Read the model definition and answer for the solid it produces. Units are mm, in the model's axes. A direction names the side the tool comes from. Round coordinates to 2 decimals unless told otherwise and drop trailing zeros. Order: outer loops, then holes, each group sorted by start corner. A loop starts at its lowest first (then second) coordinate and runs counter-clockwise, first axis right, second up. Notation, with made-up numbers: (-19, -5) - (-5, -5) arc R19 cw to (-5, 20) - close; hole circle Ø5 at (45.5, 54.5). An arc over 180 degrees is marked (long way). Answer as a JSON object with one key per item and string values. Group by question number.
Q1. Given pin 1 Ø3 at (y, z) = (4.5, -9.5) entering from +X; pin 2 Ø2 at (y, z) = (3, -13) entering from +X; pin 3 Ø3 at (x, z) = (0, 0) entering from +Y, each flat-ended and moving along its own axis, determine where each tip first touches the part or whether it passes through.
Q2. A cutting plane is placed at B-B on y = 3.2. Count the separate pieces of the cut face and the enclosed holes in it, and give its area (3 significant figures).
Q3. A tool of negligible diameter and unlimited length cuts with its end or side. For faces 3 (the cylindrical face through (5.77, 2.96, 18.65)), 4 (the cylindrical face through (19.6, 3, -6.9)), 5 (the cylindrical face through (12.32, 3.04, -16.78)), from which of +Z, -Z, +X, -X, +Y, -Y can it reach the whole face along a straight path? Write none if from no direction.
Q4. The mould has two halves that part along X. Classify faces 1 (the flat face through (6, 3, -28)), 2 (the cylindrical face through (11.046, 3.042, 17.717)): pulls with the +X half, pulls with the -X half, needs draft (parallel to the pull), parting line crosses it, or undercut.
Q5. Consider line 1 (Z direction, x = 0, y = 3); line 2 (Z direction, x = 21, y = 4.7); line 3 (X direction, y = 4.1, z = 0). Determine where each line is inside the solid, lowest interval first.
Q6. A cutting plane is placed at C-C on z = -23.5. Determine the outline of the cut face in (x, y), and give its area (3 significant figures).
Q7. A cutting plane is placed at A-A on x = 0. Determine the outline of the cut face in (y, z), and give its area (3 significant figures).
```python
from build123d import *

# Parameters (mm, degrees)
BOSS_EXTRUDE1_DEPTH = 6
BOSS_EXTRUDE2_DEPTH = 6
SKETCH2_R           = 2
CUT_EXTRUDE1_DEPTH  = 7


with BuildPart() as part:
    # Sketch1 → Boss-Extrude1 (new body)
    with BuildSketch(Plane(origin=(0, 0, 0), x_dir=(1, 0, 0), z_dir=(0, 1, 0))):
        with BuildLine():
            Line((5.999994922, -17.000000726), (6.000000976, 32.999999274))
            ThreePointArc((6.000000976, 32.999999274), (3.1827e-05, 38.999972559), (-5.999944142, 33.000006094))
            Line((-5.999944142, 33.000006094), (-5.999994922, -16.999993906))
            ThreePointArc((-5.999994922, -16.999993906), (-3.41e-06, -22.999994922), (5.999994922, -17.000000726))
        make_face()
    extrude(amount=BOSS_EXTRUDE1_DEPTH)

    # Sketch4 → Boss-Extrude2 (add)
    with BuildSketch(Plane(origin=(0, 6, 0), x_dir=(1, 0, 0), z_dir=(0, 1, 0))):
        with BuildLine():
            Line((-2.743025532, 18.19970901), (3.351302477, -22.235567688))
            ThreePointArc((3.351302477, -22.235567688), (3.541272199, -22.468242769), (3.739439393, -22.693977021))
            ThreePointArc((3.739439393, -22.693977021), (4.275797924, -22.599060868), (4.809758376, -22.491470036))
            ThreePointArc((4.809758376, -22.491470036), (5.335701359, -20.15196829), (5.179210857, -17.759188492))
            ThreePointArc((5.179210857, -17.759188492), (6.10970176, -17.460943428), (7.023146788, -17.113982885))
            ThreePointArc((7.023146788, -17.113982885), (8.392641943, -19.082324182), (10.262473747, -20.583528186))
            ThreePointArc((10.262473747, -20.583528186), (10.747026347, -20.334734439), (11.225551479, -20.074535959))
            ThreePointArc((11.225551479, -20.074535959), (11.038548046, -17.683947297), (10.183725752, -15.443598376))
            ThreePointArc((10.183725752, -15.443598376), (10.984968279, -14.884336496), (11.755563092, -14.283547788))
            ThreePointArc((11.755563092, -14.283547788), (13.644394202, -15.760775419), (15.873642273, -16.644142542))
            ThreePointArc((15.873642273, -16.644142542), (16.263334316, -16.263577617), (16.643905071, -15.873891267))
            ThreePointArc((16.643905071, -15.873891267), (15.760571298, -13.644629981), (14.283371923, -11.755776772))
            ThreePointArc((14.283371923, -11.755776772), (14.884172159, -10.985190947), (15.443446026, -10.183956787))
            ThreePointArc((15.443446026, -10.183956787), (17.683782158, -11.038812596), (20.074368023, -11.225851792))
            ThreePointArc((20.074368023, -11.225851792), (20.334573661, -10.747330553), (20.583374658, -10.262781675))
            ThreePointArc((20.583374658, -10.262781675), (19.082198626, -8.392927413), (17.113877817, -7.023402811))
            ThreePointArc((17.113877817, -7.023402811), (17.460852025, -6.109962974), (17.759111009, -5.179476534))
            ThreePointArc((17.759111009, -5.179476534), (20.151888466, -5.336002831), (22.491398079, -4.810094847))
            ThreePointArc((22.491398079, -4.810094847), (22.5989969, -4.276136005), (22.693921077, -3.739778893))
            ThreePointArc((22.693921077, -3.739778893), (20.708288865, -2.395476413), (18.423740564, -1.66696869))
            ThreePointArc((18.423740564, -1.66696869), (18.486058563, -0.691837978), (18.496801044, 0.285222939))
            ThreePointArc((18.496801044, 0.285222939), (20.829411048, 0.840934203), (22.909968714, 2.033060135))
            ThreePointArc((22.909968714, 2.033060135), (22.855400089, 2.575011992), (22.788013017, 3.115519655))
            ThreePointArc((22.788013017, 3.115519655), (20.494356761, 3.814823179), (18.096573111, 3.837582915))
            ThreePointArc((18.096573111, 3.837582915), (17.868697673, 4.787759858), (17.590969135, 5.724579102))
            ThreePointArc((17.590969135, 5.724579102), (19.656149051, 6.943150542), (21.29288809, 8.695568802))
            ThreePointArc((21.29288809, 8.695568802), (21.081000682, 9.197358874), (20.857289998, 9.69399061))
            ThreePointArc((20.857289998, 9.69399061), (18.459411122, 9.686158991), (16.161445721, 9.001148437))
            ThreePointArc((16.161445721, 9.001148437), (15.66362458, 9.84194422), (15.122102421, 10.65528129))
            ThreePointArc((15.122102421, 10.65528129), (16.73635195, 12.428437486), (17.783840917, 14.58543802))
            ThreePointArc((17.783840917, 14.58543802), (17.433461851, 15.002480058), (17.073305232, 15.411107957))
            ThreePointArc((17.073305232, 15.411107957), (14.784265796, 14.696837069), (12.790302956, 13.36492242))
            ThreePointArc((12.790302956, 13.36492242), (12.066769703, 14.021628648), (11.309570545, 14.639214975))
            ThreePointArc((11.309570545, 14.639214975), (12.329456533, 16.809403218), (12.694621435, 19.179327064))
            ThreePointArc((12.694621435, 19.179327064), (12.23688343, 19.474565051), (11.77228237, 19.758880732))
            ThreePointArc((11.77228237, 19.758880732), (9.795473575, 18.401636677), (8.282685644, 16.541164395))
            ThreePointArc((8.282685644, 16.541164395), (7.397729384, 16.955429837), (6.492133694, 17.322390167))
            ThreePointArc((6.492133694, 17.322390167), (6.827034796, 19.696779708), (6.477429129, 22.069048731))
            ThreePointArc((6.477429129, 22.069048731), (5.953004215, 22.216249477), (5.425240559, 22.350990244))
            ThreePointArc((5.425240559, 22.350990244), (3.912805358, 20.430687649), (3.017264913, 18.156258137))
            ThreePointArc((3.017264913, 18.156258137), (0.138830127, 18.404736437), (-2.743025532, 18.19970901))
        make_face()
    extrude(amount=-BOSS_EXTRUDE2_DEPTH)

    # Sketch2 → Cut-Extrude1 (cut, through all)
    with BuildSketch(Plane(origin=(0, 6, 0), x_dir=(1, 0, 0), z_dir=(0, 1, 0))):
        Circle(SKETCH2_R)
        with Locations((0, 33)):
            Circle(SKETCH2_R)
    extrude(amount=-CUT_EXTRUDE1_DEPTH, mode=Mode.SUBTRACT)


solid = part.part
```
Result set:
{
 "1": {"pin 1": "stops at x = 21.29", "pin 2": "stops at x = 17.57", "pin 3": "passes through"},
 "2": {"separate pieces": "1", "enclosed holes": "2", "area": "1,110 mm²"},
 "3": {"face 3": "+Z, +Y, -Y", "face 4": "+X, +Y, -Y", "face 5": "+Y, -Y"},
 "4": {"face 1": "pulls with the +X half", "face 2": "undercut"},
 "5": {"line 1": "z = -39 to -35, -31 to -2, 2 to 23", "line 2": "z = -9.38 to -8.3, -3.72 to -0.91, 2.54 to 5.23", "line 3": "x = -6 to -2, 2 to 18.5"},
 "6": {"outline": "(-6, 0) - (6, 0) - (6, 6) - (-6, 6) - close", "area": "72.0 mm²"},
 "7": {"outline": "(0, -39) - (6, -39) - (6, -35) - (0, -35) - close; (0, -31) - (6, -31) - (6, -2) - (0, -2) - close; (0, 2) - (6, 2) - (6, 23) - (0, 23) - close", "area": "324 mm²"}
}
